Can you work these out from the model? Positions are in its coordinate system, mm. A direction names the side the tool comes from. Round coordinates to 2 decimals unless told otherwise and drop trailing zeros. Loops run counter-clockwise (first coordinate to the right, second up) from the corner with the lowest first, then second, coordinate; pieces in that order, holes last. Notation, with made-up numbers: M 66.5,54 L 73.5,54 A20 cw 73.5,84 Z; hole C 33.5,18.5 d2. An arc over 180 degrees is marked long. Return JSON: item names as keys, results as strings.
```python
from build123d import *

# Parameters (mm, degrees)
CROQUIS1_R                                           = 15
SALIENTE_EXTRUIR1_DEPTH                              = 10
CROQUIS2_R                                           = 40
CROQUIS2_R_2                                         = 15
SALIENTE_EXTRUIR2_DEPTH                              = 10
CROQUIS3_R                                           = 40
CROQUIS3_R_2                                         = 30
SALIENTE_EXTRUIR3_DEPTH                              = 35
REFRENTADO_PARA_TORNILLO_CON_CABEZA_TRON_D           = 3.4
REFRENTADO_PARA_TORNILLO_CON_CABEZA_TRON_CBORE_D     = 7
REFRENTADO_PARA_TORNILLO_CON_CABEZA_TRON_CBORE_DEPTH = 2.4
SALIENTE_EXTRUIR4_START                              = -45
SALIENTE_EXTRUIR4_DEPTH                              = 45
REDONDEO1_R                                          = 15
CORTAR_BARRER4_PROFILE_R                             = 15


with BuildPart() as part:
    # Croquis1 → Saliente-Extruir1 (new, symmetric)
    with BuildSketch(Plane(origin=(0, 0, 0), x_dir=(0, 0, -1), z_dir=(1, 0, 0))):
        with BuildLine():
            ThreePointArc((-29.895833333, -2.497828918), (30, 0), (-29.895833333, 2.497828918))
            ThreePointArc((-29.895833333, 2.497828918), (-32.5, 0), (-29.895833333, -2.497828918))
        make_face()
        Circle(CROQUIS1_R, mode=Mode.SUBTRACT)
    extrude(amount=SALIENTE_EXTRUIR1_DEPTH, both=True)

    # Croquis2 → Saliente-Extruir2 (add)
    with BuildSketch(Plane(origin=(10, 0, 0), x_dir=(0, 0, -1), z_dir=(1, 0, 0))):
        Circle(CROQUIS2_R)
        Circle(CROQUIS2_R_2, mode=Mode.SUBTRACT)
    extrude(amount=SALIENTE_EXTRUIR2_DEPTH)

    # Croquis3 → Saliente-Extruir3 (add)
    with BuildSketch(Plane(origin=(20, 0, 0), x_dir=(0, 0, -1), z_dir=(1, 0, 0))):
        Circle(CROQUIS3_R)
        Circle(CROQUIS3_R_2, mode=Mode.SUBTRACT)
    extrude(amount=SALIENTE_EXTRUIR3_DEPTH)

    # Refrentado para tornillo con cabeza troncocónica de M31 (through all)
    with Locations(Plane.ZY.offset(-10)):
        with Locations((0, 34.5), (29.877876431, 17.25), (29.877876431, -17.25), (0, -34.5), (-29.877876431, -17.25), (-29.877876431, 17.25)):
            CounterBoreHole(REFRENTADO_PARA_TORNILLO_CON_CABEZA_TRON_D / 2, REFRENTADO_PARA_TORNILLO_CON_CABEZA_TRON_CBORE_D / 2, REFRENTADO_PARA_TORNILLO_CON_CABEZA_TRON_CBORE_DEPTH)

    # Croquis8 → Saliente-Extruir4 (add)
    with BuildSketch(Plane(origin=(55, 0, 0), x_dir=(0, 0, -1), z_dir=(1, 0, 0)).offset(SALIENTE_EXTRUIR4_START)):
        with BuildLine():
            Line((55, 20), (34.641016151, 20))
            ThreePointArc((34.641016151, 20), (40, 0), (34.641016151, -20))
            Line((34.641016151, -20), (55, -20))
            ThreePointArc((55, -20), (75, 0), (55, 20))
        make_face()
    extrude(amount=SALIENTE_EXTRUIR4_DEPTH)

    # Redondeo1
    redondeo1_edges = [part.edges().sort_by_distance(p)[0] for p in [
        (10, 0, -75),
        (10, -20, -44.820508076),
        (10, 20, -44.820508076),
    ]]
    fillet(redondeo1_edges, radius=REDONDEO1_R)

    # Cortar-Barrer4: sweep along a path in Croquis17
    with BuildLine(Plane(origin=(0, 0, 0), x_dir=(1, 0, 0), z_dir=(0, 1, 0))) as cortar_barrer4_path:
        Line((55, 55), (45, 55))
        ThreePointArc((45, 55), (34.393398282, 50.606601718), (30, 40))
        Line((30, 40), (30, 0))
    # Cortar-Barrer4 profile (on start of the path) → Cortar-Barrer4 (sweep, cut)
    with BuildSketch(Plane(origin=(55, 0, -55), x_dir=(0, 0, -1), z_dir=(-1, 0, 0))):
        Circle(CORTAR_BARRER4_PROFILE_R)
    sweep(path=cortar_barrer4_path.line, mode=Mode.SUBTRACT)

    # Redondeo2: read off the stored shape, not the designer's step
    # Redondeo2 outline → Redondeo2 (revolve, cut)
    with BuildSketch(Plane.YX):
        with BuildLine():
            ThreePointArc((15, 10), (17.928933196, 17.071068819), (25.00000285, 20))
            Line((25.00000285, 20), (15, 20))
            Line((15, 20), (15, 10))
        make_face()
    revolve(axis=Axis((0, 0, 0), (1, 0, 0)), mode=Mode.SUBTRACT)


solid = part.part
```
Q1. Suppose I cut it at C-C, the plane x = -2. Please give me the cut outline in (y, z), plus the area to 3 significant figures.
Results:
{"outline": "M -2.5,29.9 A30 ccw long 2.5,29.9 A2.5 ccw long Z; hole C 0,0 d30", "area": "2,130 mm2"}
Q2. Thinking about a two-plate mould opening in X: for faces 1 (the flat face through (40, 20, -45)), 2 (the cylindrical face through (16.144, 5.745, -30.539)), 3 (the flat face through (12.4, 18, -28)), which applies, pulls with the +X half, pulls with the -X half, needs draft (parallel to the pull), parting line crosses it, or undercut?
Results:
{"face 1": "needs draft", "face 2": "undercut", "face 3": "pulls with the -X half"}
Q3. If I drill on line 1 along Y through (x, z) = (23.5, 0); line 2 along Y through (x, z) = (50, -55); line 3 along Z through (x, y) = (37, 16), over which ranges is the centre line in solid material (lowest first)?
Results:
{"line 1": "y = -40 to -36.2, -32.8 to -30, 30 to 32.8, 36.2 to 40", "line 2": "y = -20 to -15, 15 to 20", "line 3": "z = -67 to -31.03, -28.73 to -25.38, 25.38 to 28.73, 31.03 to 36.66"}
Q4. Suppose I cut it at B-B, the plane y = 34.5. Please give me the cut outline in (x, z).
Results:
{"outline": "M 10,-20.24 L 55,-20.24 L 55,-1.7 L 12.4,-1.7 L 12.4,-3.5 L 10,-3.5 Z; M 10,3.5 L 12.4,3.5 L 12.4,1.7 L 55,1.7 L 55,20.24 L 10,20.24 Z"}
Q5. On a 3-axis mill with a long thin cutter (end or side, diameter ignored), from which of +Z, -Z, +X, -X, +Y, -Y can I reach the whole of each face in a straight line? I mean faces 4 (the cylindrical face through (49.93, -0.66, -40.015)), 5 (the cylindrical face through (40, 0, -75)), 6 (the cylindrical face through (11.183, -14.299, -27.996)), 7 (the cylindrical face through (14.51, 15.72, -44.68)), 8 (the cylindrical face through (33.998, 17.761, 28.256)). Say none if no direction works.
Results:
{"face 4": "+X", "face 5": "-Z, +X, -X", "face 6": "-X", "face 7": "-Z, -X, +Y", "face 8": "+X, -X"}
Q6. Suppose I cut it at A-A, the plane z = 0. State how many separate pieces and enclosed holes the cut face has, plus the area to 3 significant figures.
Results:
{"separate pieces": "4", "enclosed holes": "0", "area": "1,430 mm2"}
Q7. I'm going to push flat-ended pins straight in: pin 1 Ø5.5 at (y, z) = (17.25, 29.88) entering from -X; pin 2 Ø7.5 at (y, z) = (18.5, 30.5) entering from -X; pin 3 Ø2 at (y, z) = (17.25, -29.88) entering from -X; pin 4 Ø10 at (x, z) = (47, -48) entering from -Y. Where does each tip first touch, or does it pass through?
Results:
{"pin 1": "stops at x = 12.4", "pin 2": "stops at x = 10", "pin 3": "passes through", "pin 4": "stops at y = -20"}
